The model under review builds one solid part; all positions refer to its coordinate system, in mm. Face numbers are marked on the shaded views. A direction names the side the tool comes from. Round coordinates to 2 decimals unless told otherwise and drop trailing zeros. Loops run counter-clockwise (first coordinate to the right, second up) from the corner with the lowest first, then second, coordinate; pieces in that order, holes last. Notation, with made-up numbers: M 88,8.5 L 138,8.5 A35 ccw 138,42.5 Z; hole C 17.25,21.25 d7. An arc over 180 degrees is marked long. Return JSON: item names as keys, results as strings. Group by question number.
Q1. To check wall thickness, follow line 1 along Y through (x, z) = (68.5, -2); line 2 along Y through (x, z) = (81, -16); line 3 along X through (y, z) = (74, 17.5). State the ranges of each line that lie inside material, in increasing order.
Q2. Draft analysis for pull direction Y (two halves, no side actions). For the marked faces 4, 5, 6 and 7, state which applies: pulls with the +Y half, pulls with the -Y half, needs draft (parallel to the pull), parting line crosses it, or undercut.
Q3. For the marked faces 1, 2 and 3, list the 3-axis set-ups (+Z, -Z, +X, -X, +Y, -Y) from which the entire face can be reached by the end or side of a thin tool; tool diameter is ignored.
Q4. Consider section A-A (z = 43). State the section outline as (x, y) points.
Q5. Consider section B-B (x = 84). State the section outline as (y, z) points, and give its area (3 significant figures).
Q6. Consider section C-C (x = 62). State the section outline as (y, z) points.
Q7. Consider section D-D (y = 98). State the section outline as (x, z) points.
Q8. Clearance check with flat-ended pins moving along their axes: pin 1 Ø2 at (y, z) = (120.5, 2) entering from +X; pin 2 Ø12 at (x, z) = (80, -1.5) entering from +Y; pin 3 Ø4 at (y, z) = (105, -14.5) entering from +X. State where each tip first meets the part, or that it passes through.
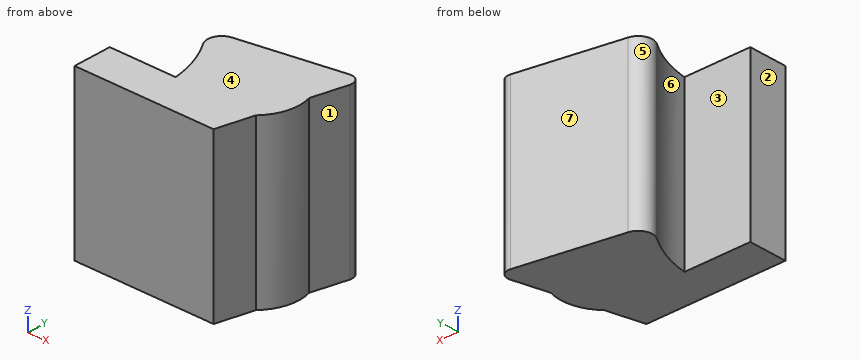
from build123d import *

# Parameters (mm, degrees)
EXTRUDE_1_DEPTH                = 50
SPLIT_BODIES_1_SURFACE_1_BACK  = 232.206
SPLIT_BODIES_1_SURFACE_1_DEPTH = 464.412
SPLIT_BODIES_1_SURFACE_2_BACK  = 232.206
SPLIT_BODIES_1_SURFACE_2_DEPTH = 464.412


with BuildPart() as part:
    # 草图2 → 凸台-拉伸1 (new, symmetric)
    with BuildSketch(Plane.XY):
        with BuildLine():
            Line((120.381757685, 62.513778912), (136.603924057, 62.513778912))
            Line((136.603924057, 62.513778912), (142.075022588, 84.611982407))
            ThreePointArc((142.075022588, 84.611982407), (149.356663913, 97.416787069), (148.890397999, 112.139827479))
            Line((148.890397999, 112.139827479), (154.115877694, 133.245956899))
            ThreePointArc((154.115877694, 133.245956899), (152.763547037, 138.423832473), (147.681959543, 140.102123925))
            Line((147.681959543, 140.102123925), (86.373837206, 128.997923897))
            ThreePointArc((86.373837206, 128.997923897), (80.146286191, 124.032461274), (80.863683371, 116.100024575))
            ThreePointArc((80.863683371, 116.100024575), (88.300101913, 101.512259026), (92.288223879, 85.631512581))
            Line((92.288223879, 85.631512581), (52.259104564, 85.631512581))
            Line((52.259104564, 85.631512581), (52.259104564, 37.347972633))
            Line((52.259104564, 37.347972633), (26.12059868, 28.530814049))
            Line((26.12059868, 28.530814049), (0, 28.530814049))
            Line((0, 28.530814049), (0, 0))
            Line((0, 0), (140.98, 0))
            Line((140.98, 0), (131.928221984, 26.834036233))
            Line((131.928221984, 26.834036233), (115.249995775, 26.834036233))
            Line((115.249995775, 26.834036233), (120.381757685, 62.513778912))
        make_face()
    extrude(amount=EXTRUDE_1_DEPTH, both=True)


with BuildPart() as body_2:
    # Split Bodies 1: the piece behind the surface
    add(part.part)
    # Split Bodies 1 surface: a surface, the sketch's curves swept straight by 464.412 mm
    with BuildLine(Plane.XY.offset(50).offset(-SPLIT_BODIES_1_SURFACE_1_BACK), mode=Mode.PRIVATE) as split_bodies_1_surface_1_path:
        Line((120.381757685, 62.513778912), (52.259104564, 62.513778912))
    split_bodies_1_surface_1 = Shell.extrude(split_bodies_1_surface_1_path.wire(), (0 * SPLIT_BODIES_1_SURFACE_1_DEPTH, 0 * SPLIT_BODIES_1_SURFACE_1_DEPTH, 1 * SPLIT_BODIES_1_SURFACE_1_DEPTH))
    split(bisect_by=split_bodies_1_surface_1, keep=Keep.BOTTOM)


with BuildPart() as part_1:
    add(part.part)

    # Split Bodies 1: split by a surface, the side it looks to stays
    # Split Bodies 1 surface: a surface, the sketch's curves swept straight by 464.412 mm
    with BuildLine(Plane.XY.offset(50).offset(-SPLIT_BODIES_1_SURFACE_2_BACK), mode=Mode.PRIVATE) as split_bodies_1_surface_2_path:
        Line((120.381757685, 62.513778912), (52.259104564, 62.513778912))
    split_bodies_1_surface_2 = Shell.extrude(split_bodies_1_surface_2_path.wire(), (0 * SPLIT_BODIES_1_SURFACE_2_DEPTH, 0 * SPLIT_BODIES_1_SURFACE_2_DEPTH, 1 * SPLIT_BODIES_1_SURFACE_2_DEPTH))
    split(bisect_by=split_bodies_1_surface_2, keep=Keep.TOP)


solid = body_2.part
Values:
{
 "1": {"line 1": "y = 62.51 to 85.63", "line 2": "y = 62.51 to 85.63, 115.89 to 125.56", "line 3": "x = 52.26 to 139.45"},
 "2": {"face 4": "needs draft", "face 5": "undercut", "face 6": "undercut", "face 7": "pulls with the +Y half"},
 "3": {"face 1": "+Z, -Z, +X", "face 2": "+Z, -Z, -X, +Y, -Y", "face 3": "+Z, -Z, -X"},
 "4": {"outline": "M 52.26,62.51 L 136.6,62.51 L 142.08,84.61 A27.18 ccw 148.89,112.14 L 154.12,133.25 A5.6 ccw 147.68,140.1 L 86.37,129 A8.4 ccw 80.86,116.1 A72.8 cw 92.29,85.63 L 52.26,85.63 Z"},
 "5": {"outline": "M 62.51,-50 L 85.63,-50 L 85.63,50 L 62.51,50 Z; M 110.9,-50 L 128.19,-50 L 128.19,50 L 110.9,50 Z", "area": "4,040 mm2"},
 "6": {"outline": "M 62.51,-50 L 85.63,-50 L 85.63,50 L 62.51,50 Z"},
 "7": {"outline": "M 89.52,-50 L 149.49,-50 L 149.49,50 L 89.52,50 Z"},
 "8": {"pin 1": "stops at x = 151.21", "pin 2": "stops at y = 128.92", "pin 3": "stops at x = 150.15"}
}
